Input: dimensioned drawing with shaded views. Units: mm. Origin: part minimum x, y, z. A direction names the side the tool comes from. Coordinates: 2 decimals unless noted, no trailing zeros. Order: outer loops, then holes, each group sorted by start corner. A loop starts at its lowest first (then second) coordinate and runs counter-clockwise, first axis right, second up.
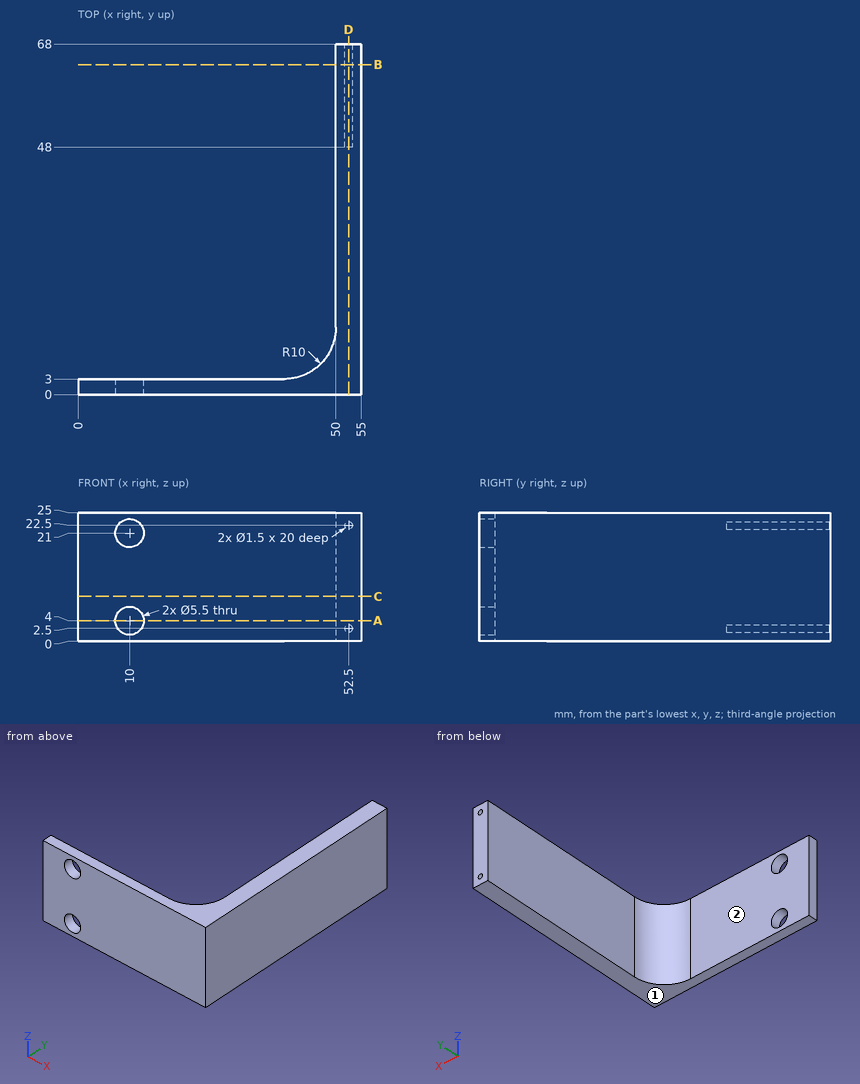
1. Section query B-B on y = 64. Return loops of the section in (x, z), plus the area to 3 significant figures.
Findings:
outline: (50, 0) - (55, 0) - (55, 25) - (50, 25) - close; hole circle Ø1.5 at (52.5, 2.5); hole circle Ø1.5 at (52.5, 22.5)
area: 121 mm2
2. Section query A-A on z = 4. Return loops of the section in (x, y), plus the area to 3 significant figures.
Findings:
outline: (0, 0) - (7.25, 0) - (7.25, 3) - (0, 3) - close; (12.75, 0) - (55, 0) - (55, 68) - (50, 68) - (50, 13) arc R10 cw to (40, 3) - (12.75, 3) - close
area: 495 mm2
3. Ray query, line 1 (Z direction, x = 10, y = 1.25); line 2 (X direction, y = 54.75, z = 22.5); line 3 (Z direction, x = 52.5, y = 57). Return the intervals inside material, ascending.
Findings:
line 1: z = 0 to 1.25, 6.75 to 18.25, 23.75 to 25
line 2: x = 50 to 51.75, 53.25 to 55
line 3: z = 0 to 1.75, 3.25 to 21.75, 23.25 to 25
4. Section query D-D on x = 52.5. Return loops of the section in (y, z).
Findings:
outline: (0, 0) - (68, 0) - (68, 1.75) - (48, 1.75) - (48, 3.25) - (68, 3.25) - (68, 21.75) - (48, 21.75) - (48, 23.25) - (68, 23.25) - (68, 25) - (0, 25) - close
5. Section query C-C on z = 8.75. Return loops of the section in (x, y), plus the area to 3 significant figures.
Findings:
outline: (0, 0) - (55, 0) - (55, 68) - (50, 68) - (50, 13) arc R10 cw to (40, 3) - (0, 3) - close
area: 511 mm2
6. Pin query (flat end, axial travel): P1, Ø4, axis at x = 29.5, z = 9, coming from the +Y side; P2, Ø12, axis at x = 40.5, z = 13, coming from the -Y side; P3, Ø1.5, axis at x = 41, z = 8.5, coming from the +Y side; P4, Ø1.2, axis at x = 52.5, z = 2.5, coming from the +Y side. Return the tip coordinate at first contact, or that it passes through.
Findings:
P1: stops at y = 3
P2: stops at y = 0
P3: stops at y = 3.15
P4: stops at y = 48
7. Access query for the marked faces 1 and 2. Directions: +Z, -Z, +X, -X, +Y, -Y. A direction counts if a zero-diameter tool reaches every point of the face in a straight line with its end or side. Return the directions, or none.
Findings:
face 1: -Z, +X, -X, +Y, -Y
face 2: +Z, -Z, -X, +Y
